Drawing for the job (mm, zero at the part's lowest x, y, z). A direction names the side the tool comes from. Give positions to 0.01 mm unless a question says otherwise; leave off trailing zeros. Loops run counter-clockwise (first coordinate to the right, second up) from the corner with the lowest first, then second, coordinate; pieces in that order, holes last.
1) Wall check: line 1 (Z direction, x = 2.95, y = 19); line 2 (Z direction, x = 0.6, y = 2.75); line 3 (Y direction, x = 4.35, z = 15). Give the ranges that are in metal, low to high.
2) 3-axis set-ups, long thin cutter, end or side, ignore diameter. For the marked faces 1, 2, 3, 4 and 5: which of +Z, -Z, +X, -X, +Y, -Y reach the whole face in a straight line?
3) Band-saw the part on D-D on z = 30.5. List the corners of the cut face in (x, y), then the cut area to 3 significant figures.
4) Band-saw the part on A-A on y = 19. List the corners of the cut face in (x, z), then the cut area to 3 significant figures.
5) Band-saw the part on B-B on x = 0.95. List the corners of the cut face in (y, z).
6) Flat gauge pins, fed straight in: P1, Ø1.5, axis at y = 5, z = 16, coming from the +X side; P2, Ø3, axis at x = 4, y = 3, coming from the -Z side; P3, Ø6.5, axis at y = 19, z = 27.5, coming from the +X side; P4, Ø1.8, axis at x = 2, z = 19, coming from the -Y side. Where does each tip first touch, or does it go through?
7) Band-saw the part on C-C on z = 7.5. List the corners of the cut face in (x, y), then the cut area to 3 significant figures.
8) Two-plate mould, pull along Z, no slides. Class the marked faces 6, 7, 8 and 9: +Z half, -Z half, draft (parallel to the pull), parting line (faces both ways), or undercut.
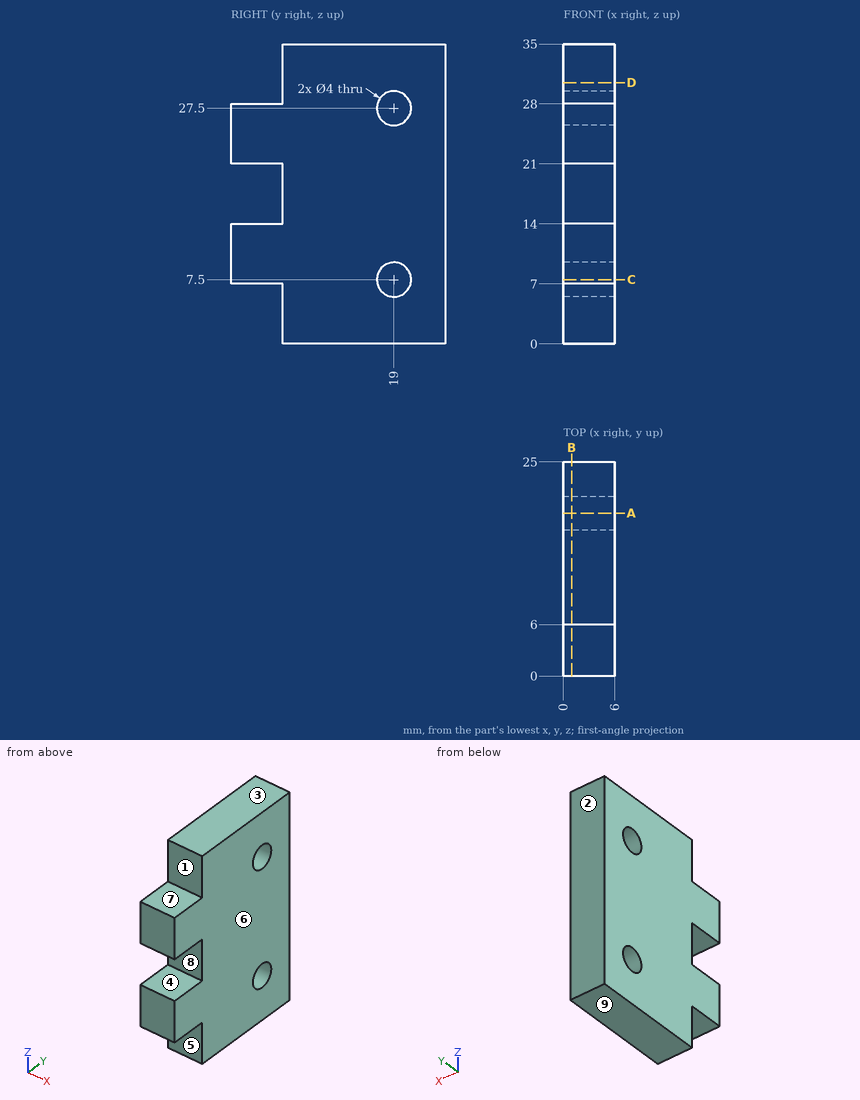
Findings below:
1. line 1: z = 0 to 5.5, 9.5 to 25.5, 29.5 to 35
1. line 2: z = 7 to 14, 21 to 28
1. line 3: y = 6 to 25
2. face 1: +Z, +X, -X, -Y
2. face 2: +Z, -Z, +X, -X, +Y
2. face 3: +Z, +X, -X, +Y, -Y
2. face 4: +X, -X, -Y
2. face 5: -Z, +X, -X, -Y
3. outline: (0, 6) - (6, 6) - (6, 25) - (0, 25) - close
3. area: 114 mm2
4. outline: (0, 0) - (6, 0) - (6, 5.5) - (0, 5.5) - close; (0, 9.5) - (6, 9.5) - (6, 25.5) - (0, 25.5) - close; (0, 29.5) - (6, 29.5) - (6, 35) - (0, 35) - close
4. area: 162 mm2
5. outline: (0, 7) - (6, 7) - (6, 0) - (25, 0) - (25, 35) - (6, 35) - (6, 28) - (0, 28) - (0, 21) - (6, 21) - (6, 14) - (0, 14) - close; hole circle Ø4 at (19, 7.5); hole circle Ø4 at (19, 27.5)
6. P1: passes through
6. P2: stops at z = 7
6. P3: stops at x = 6
6. P4: stops at y = 6
7. outline: (0, 0) - (6, 0) - (6, 17) - (0, 17) - close; (0, 21) - (6, 21) - (6, 25) - (0, 25) - close
7. area: 126 mm2
8. face 6: draft
8. face 7: +Z half
8. face 8: undercut
8. face 9: -Z half
